```python
from build123d import *

# Parameters (mm, degrees)
BOSS_EXTRUDE3_DEPTH      = 75
BOSS_EXTRUDE4_DEPTH      = 100
BOSS_EXTRUDE4_DEPTH_BACK = 216.481457


with BuildPart() as part:
    # Sketch1 → Boss-Extrude3 (new body)
    with BuildSketch(Plane(origin=(0, 0, 0), x_dir=(1, 0, 0), z_dir=(0, 1, 0))):
        with BuildLine():
            ThreePointArc((-70.710678119, -70.710678119), (100, 0), (-70.710678119, 70.710678119))
            ThreePointArc((-70.710678119, 70.710678119), (-85.125192843, 63.602226114), (-100.888347648, 66.737712554))
            ThreePointArc((-100.888347648, 66.737712554), (-216.481456572, 0), (-100.888347648, -66.737712554))
            ThreePointArc((-100.888347648, -66.737712554), (-85.125192843, -63.602226114), (-70.710678119, -70.710678119))
        make_face()
    extrude(amount=-BOSS_EXTRUDE3_DEPTH)

    # Sketch6 → Boss-Extrude4 (add, two sides)
    with BuildSketch(Plane(origin=(0, 0, 0), x_dir=(0, 0, -1), z_dir=(1, 0, 0))) as boss_extrude4_sk:
        with BuildLine():
            Line((20, 0), (20, 11.326222077))
            ThreePointArc((20, 11.326222077), (0, 12.171), (-20, 11.326222077))
            Line((-20, 11.326222077), (-20, 0))
            Line((-20, 0), (20, 0))
        make_face()
    extrude(amount=BOSS_EXTRUDE4_DEPTH)
    extrude(boss_extrude4_sk.sketch, amount=-BOSS_EXTRUDE4_DEPTH_BACK)


solid = part.part
```
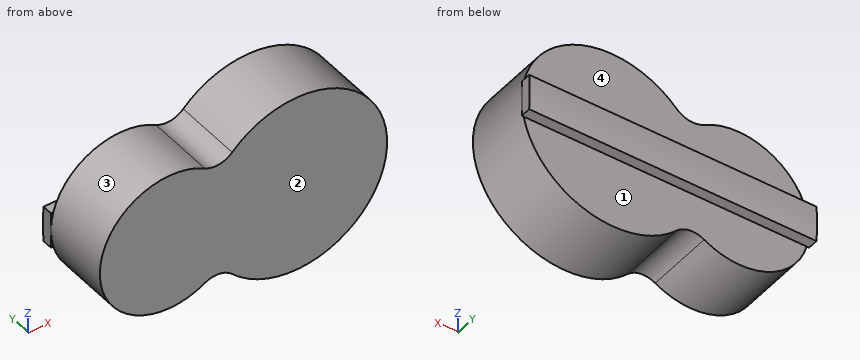
CAD build for the part. Positions are in the model's coordinates, mm. Face numbers are marked on the shaded views. A direction names the side the tool comes from. Round coordinates to 2 decimals unless told otherwise and drop trailing zeros. Write each loop counter-clockwise with the first axis right and the second up, starting at its lowest first coordinate (ties: lowest second). Pieces come first, ordered by that corner, then holes. Notation, with made-up numbers: M -21,22.25 L 11,22.25 A11 cw 11,43.25 Z; hole C 26,50 d4. An arc over 180 degrees is marked long. One line per question, with ' | ' between items.
1. Cut at C-C on y = -13. Write the cut outline in (x, z).
Working result:
outline: M -100.89,-66.74 A25 cw -70.71,-70.71 A100 ccw long -70.71,70.71 A25 cw -100.89,66.74 A77.06 ccw long Z
2. Which spindle directions (+Z, -Z, +X, -X, +Y, -Y) get a long thin tool onto all of the face, cutting with end or side? Do the marked faces 1 and 2. Say none if no direction does.
Working result:
face 1: -Z, +X, -X, +Y | face 2: +Z, -Z, +X, -X, -Y
3. Cut at A-A on x = 0. Write the cut outline in (y, z), and give its area (3 significant figures).
Working result:
outline: M -75,-100 L 0,-100 L 0,-20 L 11.33,-20 A237.17 ccw 11.33,20 L 0,20 L 0,100 L -75,100 Z | area: 15,500 mm2
4. Cut at D-D on z = -25.5. Write the cut outline in (x, y), and give its area (3 significant figures).
Working result:
outline: M -212.14,-75 L 96.69,-75 L 96.69,0 L -212.14,0 Z | area: 23,200 mm2
5. Probe L1, parallel to Z at x = -38, y = 5.5; L2, parallel to Y at x = -21, z = -71; L3, parallel to Z at x = -87.5, y = -8.5. List the from-to ranges inside material, lowest first. Write a range as from..to.
Working result:
L1: -20..20 | L2: -75..0 | L3: -63.4..63.4
6. Cut at B-B on z = 16.5. Write the cut outline in (x, y), and give its area (3 significant figures).
Working result:
outline: M -216.48,0 L -214.69,0 L -214.69,-75 L 98.63,-75 L 98.63,0 L 100,0 L 100,11.6 L -216.48,11.6 Z | area: 27,200 mm2
7. Mould opens along X. For the marked faces 3 and 4 say: pulls with the +X half, pulls with the -X half, needs draft (parallel to the pull), parting line crosses it, or undercut.
Working result:
face 3: undercut | face 4: needs draft
8. Pin check, flat tips, straight feed: pin 1 Ø8 at (x, y) = (-54.5, -19) entering from -Z; pin 2 Ø6 at (x, y) = (-130, -49.5) entering from +Z; pin 3 Ø4 at (x, y) = (-91, -31.5) entering from -Z. Stop position of each tip, or through.
Working result:
pin 1: z = -86.31 | pin 2: z = 76.79 | pin 3: z = -63.82
